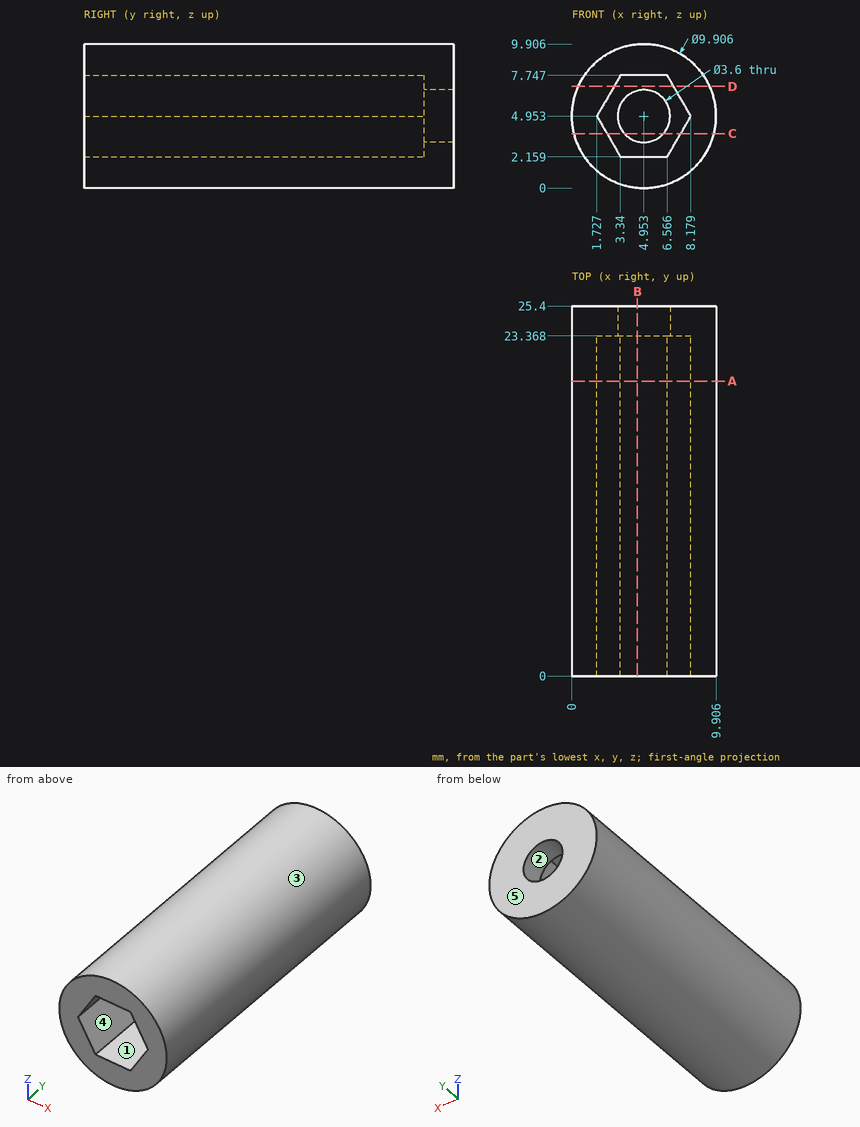
Source: three-view drawing plus pictorial views. Frame: mm from the lowest corner of the part. A direction names the side the tool comes from. Coordinates: 2 decimals unless noted, no trailing zeros. Loops run counter-clockwise (first coordinate to the right, second up) from the corner with the lowest first, then second, coordinate; pieces in that order, holes last. Notation, with made-up numbers: (-26.5, -16.5) -> (7.5, -16.5) arc R19 cw to (7.5, 17.5) -> close; hole circle Ø1 at (19.25, -11). An arc over 180 degrees is marked (long way). Write each question's results on one line, items separated by ' | '. Start each with the question number.
Q1. Section A-A, the plane y = 20.25. Return the cut outline in (x, z).
Q2. Ray query, line 1 (Z direction, x = 5, y = 14.75); line 2 (X direction, y = 13.75, z = 5.25); line 3 (Z direction, x = 6.75, y = 22.5). Return the intervals inside material, ascending. Write a range as from..to.
Q3. Reachability of the marked faces 1 and 2 from +Z, -Z, +X, -X, +Y, -Y: full face, straight path, thin tool, end or side. Return the list, or none.
Q4. Section B-B, the plane x = 4.5. Return the cut outline in (y, z) (1 decimal).
Q5. Pin query (flat end, axial travel): pin 1 (4 mm diameter, centred on x = 3, y = 5, fed in from +Z); pin 2 (1.7 mm diameter, centred on x = 4, z = 5.5, fed in from -Y); pin 3 (1 mm diameter, centred on x = 2, y = 18.5, fed in from +Z); pin 4 (5 mm diameter, centred on x = 1.5, y = 18.5, fed in from +Z). Return the tip coordinate at first contact, or that it passes through.
Q6. Section C-C, the plane z = 3.75. Return the cut outline in (x, y) (1 decimal), plus the area to 3 significant figures.
Q7. Pull-direction query (X, two-part tool) for the marked faces 3, 4 and 5; classes: released by +X, released by -X, zero draft, split by the parting line, or undercut.
Q8. Section D-D, the plane z = 7. Return the cut outline in (x, y), plus the area to 3 significant figures.
Found:
1) outline: circle Ø9.91 at (4.95, 4.95); hole (1.73, 4.95) -> (3.34, 2.16) -> (6.57, 2.16) -> (8.18, 4.95) -> (6.57, 7.75) -> (3.34, 7.75) -> close
2) line 1: 0..2.16, 7.75..9.91 | line 2: 0.01..1.9, 8.01..9.9 | line 3: 0.34..2.48, 7.43..9.57
3) face 1: -Y | face 2: +Y, -Y
4) outline: (0, 0) -> (25.4, 0) -> (25.4, 3.2) -> (23.4, 3.2) -> (23.4, 2.2) -> (0, 2.2) -> close; (0, 7.7) -> (23.4, 7.7) -> (23.4, 6.7) -> (25.4, 6.7) -> (25.4, 9.9) -> (0, 9.9) -> close
5) pin 1: z = 9.91 | pin 2: y = 23.37 | pin 3: z = 9.26 | pin 4: z = 9.81
6) outline: (0.1, 0) -> (2.4, 0) -> (2.4, 23.4) -> (3.6, 23.4) -> (3.6, 25.4) -> (0.1, 25.4) -> close; (6.3, 23.4) -> (7.5, 23.4) -> (7.5, 0) -> (9.8, 0) -> (9.8, 25.4) -> (6.3, 25.4) -> close | area: 120 mm2
7) face 3: split by the parting line | face 4: undercut | face 5: zero draft
8) outline: (0.44, 0) -> (2.91, 0) -> (2.91, 23.37) -> (7, 23.37) -> (7, 0) -> (9.46, 0) -> (9.46, 25.4) -> (0.44, 25.4) -> close | area: 134 mm2
